Autodesk Inventor part; units mm, degrees
ref_plane "YZ Plane" through (0, 0, 0) normal (1, 0, 0) x (0, 1, 0)
ref_plane "XZ Plane" through (0, 0, 0) normal (0, 1, 0) x (-1, 0, 0)
ref_plane "XY Plane" through (0, 0, 0) normal (0, 0, 1) x (1, 0, 0)
sketch "Sketch1" plane through (0, 0, 0) normal (1, 0, 0) x (0, 1, 0)
  line L0 (0, 0) -> (76.2, 0)
  line L1 (76.2, 0) -> (76.2, 9.525)
  line L2 (76.2, 9.525) -> (9.525, 9.525)
  line L3 (0, 9.525) -> (0, 0)
  line L4 (9.525, 9.525) -> (9.525, 85.725)
  line L5 (9.525, 85.725) -> (0, 85.725)
  line L6 (0, 85.725) -> (0, 9.525)
  dimension "d4" = 76.2
  dimension "d5" = 9.525
  dimension "d6" = 9.525
  dimension "d7" = 76.2
extrude "Extrusion1" add sketch "Sketch1" along normal blind 95.25
sketch "Sketch2" plane through (0, 9.525, 85.725) normal (0, 1, 0) x (1, 0, 0)
  line L0 (95.25, 76.2) -> (95.25, 0)
  circle A0 centre (82.55, 38.1) radius 4.4901
  circle A1 centre (12.7, 38.1) radius 5.7238
  point P0 (0, 85.725)
  dimension "d13" = 12.7
  dimension "d14" = 69.85
hole "Hole1" at (12.7, 9.525, 47.625) at (82.55, 9.525, 47.625) direction (0, -1, 0) diameter 12.7 depth 25.4 tip angle 118
sketch "Sketch3" plane through (0, 9.525, 9.525) normal (0, 0, 1) x (1, 0, 0)
  line L0 (95.25, 66.675) -> (95.25, 0)
  circle A0 centre (82.55, 33.3375) radius 4.4901
  circle A1 centre (12.7, 33.3375) radius 3.5498
  point P0 (0, -9.525)
  dimension "d22" = 12.7
  dimension "d23" = 69.85
hole "Hole2" at (12.7, 42.8625, 9.525) at (82.55, 42.8625, 9.525) direction (0, 0, -1) diameter 12.7 depth 25.4 tip angle 118
properties part number "0wrab" material "Steel, Galvanized"
Verification items for the finished model (mm, model axes). A direction names the side the tool comes from. Give positions to 0.01 mm unless a question says otherwise; leave off trailing zeros. Order: outer loops, then holes, each group sorted by start corner. A loop starts at its lowest first (then second) coordinate and runs counter-clockwise, first axis right, second up. Notation, with made-up numbers: M -10,25 L 9,25 A21 cw 9,38 Z; hole C 42,-5 d9. An arc over 180 degrees is marked long. Use one line per item in the form item = value. Start each with the question number.
Q1. Section check D-D (y = 5). Enter the section's corners in (x, z) (3 decimals), then the cut area to 3 significant figures.
Q2. Access from +Z, -Z, +X, -X, +Y, -Y to the whole of each face (thin tool, end or side, straight path). Record for faces 1 (the cylindrical face through (82.27, 4.7, 41.28)), 2 (the flat face through (47, 9.525, 47)).
Q3. Section check B-B (y = 41). Enter the section's corners in (x, z) (3 decimals), then the cut area to 3 significant figures.
Q4. Scan lines: line 1 along X through (y, z) = (42.5, 6.5); line 2 along Z through (x, y) = (82.55, 4.75) (3 decimals); line 3 along X through (y, z) = (41.5, 4). Record each from-to range of solid material in increasing order. Write a range as [from, to].
Q5. Section check C-C (x = 62.5). Enter the section's corners in (y, z) (3 decimals).
Q6. Section check A-A (x = 12.7). Enter the section's corners in (y, z) (1 decimal), then the cut area to 3 significant figures.
Q7. Go/stop test with flat-tipped pins: pin 1 Ø20.5 at (x, y) = (82.55, 42.86) entering from -Z; pin 2 Ø23 at (x, z) = (27, 62.5) entering from +Y (3 decimals); pin 3 Ø20 at (x, y) = (69.5, 41) entering from +Z (3 decimals); pin 4 Ø7.5 at (x, y) = (12.7, 42.86) entering from +Z. Record where each tip stops, or that it passes through.
Q8. Mould release check, pull along Z, two halves, no side actions. Record for faces 3 (the cylindrical face through (12.42, 4.7, 41.28)), 4 (the flat face through (47, 43, 9.525)), 5 (the flat face through (47, 76.2, 5)): +Z half, -Z half, draft (parallel to the pull), parting line (faces both ways), or undercut.
Evaluation:
q1.outline = M 0,0 L 95.25,0 L 95.25,85.725 L 0,85.725 Z; hole C 12.7,47.625 d12.7; hole C 82.55,47.625 d12.7
q1.area = 7,910 mm2
q2.face_1 = +Y, -Y
q2.face_2 = +Z, +X, -X, +Y
q3.outline = M 0,0 L 6.629,0 L 6.629,9.525 L 0,9.525 Z; M 18.771,0 L 76.479,0 L 76.479,9.525 L 18.771,9.525 Z; M 88.621,0 L 95.25,0 L 95.25,9.525 L 88.621,9.525 Z
q3.area = 676 mm2
q4.line_1 = [0, 6.36], [19.04, 76.21], [88.89, 95.25]
q4.line_2 = [0, 41.275], [53.975, 85.725]
q4.line_3 = [0, 6.5], [18.9, 76.35], [88.75, 95.25]
q5.outline = M 0,0 L 76.2,0 L 76.2,9.525 L 9.525,9.525 L 9.525,85.725 L 0,85.725 Z
q6.outline = M 0,0 L 36.5,0 L 36.5,9.5 L 9.5,9.5 L 9.5,41.3 L 0,41.3 Z; M 0,54 L 9.5,54 L 9.5,85.7 L 0,85.7 Z; M 49.2,0 L 76.2,0 L 76.2,9.5 L 49.2,9.5 Z
q6.area = 1,210 mm2
q7.pin_1 = 0
q7.pin_2 = 9.525
q7.pin_3 = 9.525
q7.pin_4 = through
q8.face_3 = undercut
q8.face_4 = +Z half
q8.face_5 = draft
